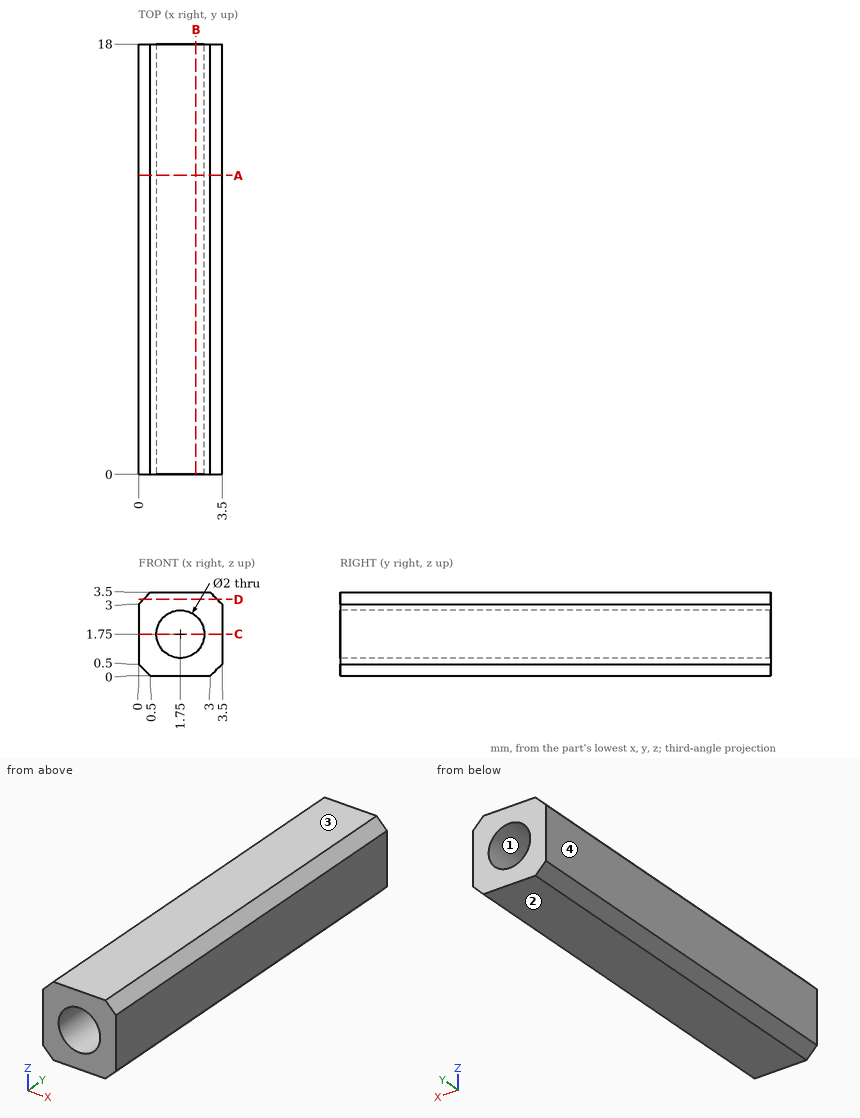
Here's the drawing with two shaded views (mm, measured from the low corner). I have some questions. Give positions to 0.01 mm unless a question says otherwise; leave off trailing zeros. Loops run counter-clockwise (first coordinate to the right, second up) from the corner with the lowest first, then second, coordinate; pieces in that order, holes last. Notation, with made-up numbers: M -10.75,-6 L 35.25,-6 A29 cw 35.25,26 Z; hole C -10.75,15 d11. An arc over 180 degrees is marked long. Use one line per item in the form item = value. Start each with the question number.
(1) Please list where these lines run through material, in increasing order: line 1 (X direction, y = 14.25, z = 1.75); line 2 (X direction, y = 5.25, z = 2.35).
(2) I want a section at D-D, the plane z = 3.2. Write out the boundary of the cut face in (x, y), and give its area (3 significant figures).
(3) I want a section at B-B, the plane x = 2.4. Write out the boundary of the cut face in (y, z).
(4) Thinking about a two-plate mould opening in Z: for the marked faces 1, 2, 3 and 4, which applies, released by +Z, released by -Z, zero draft, split by the parting line, or undercut?
(5) I'm going to push a flat-ended pin straight in: P1, Ø1.2, axis at x = 1.75, z = 1.75, coming from the -Y side. Where does the tip first touch, or does it pass through?
(6) I want a section at C-C, the plane z = 1.75. Write out the boundary of the cut face in (x, y), and give its area (3 significant figures).
(7) I want a section at A-A, the plane y = 12.5. Write out the boundary of the cut face in (x, z), and give its area (3 significant figures).
Worked out:
q1.line_1 = 0 to 0.75, 2.75 to 3.5
q1.line_2 = 0 to 0.95, 2.55 to 3.5
q2.outline = M 0.2,0 L 3.3,0 L 3.3,18 L 0.2,18 Z
q2.area = 55.8 mm²
q3.outline = M 0,0 L 18,0 L 18,0.99 L 0,0.99 Z; M 0,2.51 L 18,2.51 L 18,3.5 L 0,3.5 Z
q4.face_1 = undercut
q4.face_2 = released by -Z
q4.face_3 = released by +Z
q4.face_4 = zero draft
q5.P1 = through
q6.outline = M 0,0 L 0.75,0 L 0.75,18 L 0,18 Z; M 2.75,0 L 3.5,0 L 3.5,18 L 2.75,18 Z
q6.area = 27.0 mm²
q7.outline = M 0,0.5 L 0.5,0 L 3,0 L 3.5,0.5 L 3.5,3 L 3,3.5 L 0.5,3.5 L 0,3 Z; hole C 1.75,1.75 d2
q7.area = 8.61 mm²
